from build123d import *

# Parameters (mm, degrees)
SKETCH1_R           = 2
SKETCH1_R_2         = 1.5
BOSS_EXTRUDE1_DEPTH = 3


with BuildPart() as part:
    # Sketch1 → Boss-Extrude1 (new body)
    with BuildSketch(Plane.XY):
        with BuildLine():
            Line((-1.2291645, 7.272594351), (-33.6207003, 6.790167677))
            ThreePointArc((-33.6207003, 6.790167677), (-39.756779375, -2.600284623), (-28.692691922, -4.44907603))
            ThreePointArc((-28.692691922, -4.44907603), (-17.430920536, 0.485186112), (-6.174483245, -4.461232505))
            ThreePointArc((-6.174483245, -4.461232505), (5.388610173, -2.538681661), (-1.0207003, 7.275699134))
            Line((-1.0207003, 7.275699134), (-1.2291645, 7.272594351))
        make_face()
        with Locations((-33.6207003, 0.090167677)):
            Circle(SKETCH1_R, mode=Mode.SUBTRACT)
        with Locations((-1.0207003, 0.275699134)):
            Circle(SKETCH1_R, mode=Mode.SUBTRACT)
        with Locations((1.881986284, 4.492783471)):
            Circle(SKETCH1_R_2, mode=Mode.SUBTRACT)
    extrude(amount=BOSS_EXTRUDE1_DEPTH)


solid = part.part
CAD build for the part. Positions are in the model's coordinates, mm. Coordinates: 2 decimals unless noted, no trailing zeros. Order: outer loops, then holes, each group sorted by start corner. A loop starts at its lowest first (then second) coordinate and runs counter-clockwise, first axis right, second up.
Item 1: Band-saw the part on A-A on y = -3. List the corners of the cut face in (x, z).
Check sheet entries:
outline: (-39.57, 0) - (-27.16, 0) - (-27.16, 3) - (-39.57, 3) - close; (-7.72, 0) - (5.17, 0) - (5.17, 3) - (-7.72, 3) - close
Item 2: Band-saw the part on B-B on z = 0.6. List the corners of the cut face in (x, y), plus the area to 3 significant figures.
Check sheet entries:
outline: (-33.62, 6.79) arc R6.7 ccw (long way) to (-28.69, -4.45) arc R15.3 cw to (-6.17, -4.46) arc R7 ccw (long way) to (-1.02, 7.28) - close; hole circle Ø4 at (-33.62, 0.09); hole circle Ø4 at (-1.02, 0.28); hole circle Ø3 at (1.88, 4.49)
area: 428 mm2
Item 3: Drill centre lines: L1, parallel to X at y = -0.75, z = 1.15; L2, parallel to X at y = 1.5, z = 1.25; L3, parallel to X at y = -5.5, z = 2.15. Where is each one in solid material? Low to high.
Check sheet entries:
L1: x = -40.27 to -35.44, -31.81 to -23.46, -11.42 to -2.74, 0.7 to 5.9
L2: x = -40.17 to -35.04, -32.2 to -2.6, 0.56 to 5.87
L3: x = -37.31 to -29.93, -4.98 to 2.93
Item 4: Two-plate mould, pull along X, no slides. Class faces 1 (the face through (-17, 2, 0)), 2 (the face through (3.27, 3.92, 1.48)): +X half, -X half, draft (parallel to the pull), parting line (faces both ways), or undercut.
Check sheet entries:
face 1: draft
face 2: undercut
Item 5: Band-saw the part on C-C on x = 2. List the corners of the cut face in (y, z).
Check sheet entries:
outline: (-6.04, 0) - (3, 0) - (3, 3) - (-6.04, 3) - close; (5.99, 0) - (6.59, 0) - (6.59, 3) - (5.99, 3) - close
Item 6: Band-saw the part on D-D on y = 1.25. List the corners of the cut face in (x, z), plus the area to 3 significant figures.
Check sheet entries:
outline: (-40.22, 0) - (-35.25, 0) - (-35.25, 3) - (-40.22, 3) - close; (-31.99, 0) - (-2.77, 0) - (-2.77, 3) - (-31.99, 3) - close; (0.73, 0) - (5.91, 0) - (5.91, 3) - (0.73, 3) - close
area: 118 mm2
Item 7: Pin check, flat tips, straight feed: pin 1 Ø5 at (x, y) = (-12.5, 1) entering from -Z; pin 2 Ø1.5 at (y, z) = (1.5, 2.5) entering from +X; pin 3 Ø3.5 at (x, y) = (-33.62, 0.09) entering from +Z. Stop position of each tip, or through.
Check sheet entries:
pin 1: stops at z = 0
pin 2: stops at x = 5.96
pin 3: passes through
